Geometry: final body of the model. Coordinates: model frame, mm. A direction names the side the tool comes from. Round coordinates to 2 decimals unless told otherwise and drop trailing zeros. Write each loop counter-clockwise with the first axis right and the second up, starting at its lowest first coordinate (ties: lowest second). Pieces come first, ordered by that corner, then holes. Notation, with made-up numbers: (42, 16) -> (53, 16) arc R27 cw to (53, 47) -> close; hole circle Ø11 at (70, 84). An arc over 180 degrees is marked (long way). Use one line per item in the form item = value. Start each with the question number.
1. Draft query along Y for faces 4 (the face through (35, -37.5, 4)), 5 (the face through (68.217, 35.647, 8.098)), 6 (the face through (70, 0, 8)), 7 (the face through (35.042, -42.571, 17.802)). Return one class per face: pulls with the +Y half, pulls with the -Y half, needs draft (parallel to the pull), parting line crosses it, or undercut.
2. Line query: L1, parallel to Y at x = 27.5, z = 14.75; L2, parallel to X at y = -10, z = 4; L3, parallel to Y at x = -39, z = 13.5. Output: solid intervals per line, ascending.
3. Pin query (flat end, axial travel): pin 1 Ø6 at (x, z) = (-37, 6) entering from +Y; pin 2 Ø1.5 at (x, y) = (19, -17.5) entering from +Z; pin 3 Ø3.5 at (y, z) = (-41, 10) entering from -X; pin 4 Ø1.2 at (y, z) = (-41.5, 15) entering from -X. Return the tip coordinate at first contact, or that it passes through.
4. Cut plane B-B, the plane y = 29. Return the cut outline in (x, z), plus the area to 3 significant figures.
5. Reachability of faces 1 (the face through (-68.681, -35.883, 7.902)), 2 (the face through (1, 37, 8)), 3 (the face through (32, -40, 13)) from +Z, -Z, +X, -X, +Y, -Y: full face, straight path, thin tool, end or side. Return the list, or none.
6. Cut plane C-C, the plane x = -14. Return the cut outline in (y, z).
```python
from build123d import *

# Parameters (mm, degrees)
PAD_DEPTH            = 15
POCKET_DEPTH         = 14
SKETCH002_R          = 1
PAD001_DEPTH         = 140
SKETCH008_W          = 20
SKETCH008_H          = 20
SKETCH008_W_2        = 6
SKETCH008_W_3        = 64
POCKET004_DEPTH      = 15.001
POCKET004_DEPTH_BACK = 3.001
SKETCH009_W          = 15
SKETCH009_H          = 3.5
PAD004_DEPTH         = 1
POCKET005_DEPTH      = 140.001
CHAMFER001_SIZE      = 1


with BuildPart() as part:
    # Sketch → Pad (new body)
    with BuildSketch(Plane.XY):
        with BuildLine():
            Line((-70, 32.5), (-70, -32.5))
            ThreePointArc((-70, -32.5), (-68.535534, -36.035534), (-65, -37.5))
            Line((-65, -37.5), (65, -37.5))
            ThreePointArc((65, -37.5), (68.535534, -36.035534), (70, -32.5))
            Line((70, -32.5), (70, 32.5))
            ThreePointArc((70, 32.5), (68.535534, 36.035534), (65, 37.5))
            Line((65, 37.5), (-65, 37.5))
            ThreePointArc((-65, 37.5), (-68.535534, 36.035534), (-70, 32.5))
        make_face()
    extrude(amount=PAD_DEPTH)

    # Sketch001 (on Face10 of Pad) → Pocket (cut)
    with BuildSketch(Plane.XY.offset(15)):
        with BuildLine():
            Line((-69.5, 32.5), (-69.5, -32.5))
            ThreePointArc((-69.5, -32.5), (-68.181981, -35.681981), (-65, -37))
            Line((-65, -37), (65, -37))
            ThreePointArc((65, -37), (68.181981, -35.681981), (69.5, -32.5))
            Line((69.5, -32.5), (69.5, 32.5))
            ThreePointArc((69.5, 32.5), (68.181981, 35.681981), (65, 37))
            Line((65, 37), (-65, 37))
            ThreePointArc((-65, 37), (-68.181981, 35.681981), (-69.5, 32.5))
        make_face()
    extrude(amount=-POCKET_DEPTH, mode=Mode.SUBTRACT)

    # Sketch002 (on Face9 of Pocket) → Pad001 (join)
    with BuildSketch(Plane.YZ.offset(70)):
        with BuildLine():
            ThreePointArc((-38.5, 15), (-42.64805, 17.771639), (-43.62132, 12.87868))
            Line((-43.62132, 12.87868), (-37.5, 6.757359))
            Line((-37.5, 15), (-37.5, 6.757359))
            Line((-37.5, 15), (-38.5, 15))
        make_face()
        with Locations((-41.5, 15)):
            Circle(SKETCH002_R, mode=Mode.SUBTRACT)
    extrude(amount=-PAD001_DEPTH)

    # Sketch008 (on Face17 of Pad001) → Pocket004 (cut, two sides)
    with BuildSketch(Plane.XY.offset(15)) as pocket004_sk:
        with Locations((-60, -47.49)):
            Rectangle(SKETCH008_W, SKETCH008_H)
        with Locations((60, -47.49)):
            Rectangle(SKETCH008_W, SKETCH008_H)
        with Locations((41, -47.49)):
            Rectangle(SKETCH008_W_2, SKETCH008_H)
        with Locations((-41, -47.49)):
            Rectangle(SKETCH008_W_2, SKETCH008_H)
        with Locations((0, -47.49)):
            Rectangle(SKETCH008_W_3, SKETCH008_H)
    extrude(amount=-POCKET004_DEPTH, mode=Mode.SUBTRACT)
    extrude(pocket004_sk.sketch, amount=POCKET004_DEPTH_BACK, mode=Mode.SUBTRACT)

    # Sketch009 (on Face6 of Pocket004) → Pad004 (join)
    with BuildSketch(Plane(origin=(0, 37.5, 0), x_dir=(-1, 0, 0), z_dir=(0, 1, 0))):
        with Locations((32.5, 12.25)):
            Rectangle(SKETCH009_W, SKETCH009_H)
        with Locations((-32.5, 12.25)):
            Rectangle(SKETCH009_W, SKETCH009_H)
    extrude(amount=PAD004_DEPTH)

    # Sketch010 (on Face1 of Pad004) → Pocket005 (cut, through all)
    with BuildSketch(Plane(origin=(-70, 0, 0), x_dir=(0, -1, 0), z_dir=(-1, 0, 0))):
        Polygon((-37.5, 10.5), (-38.5, 11.5), (-38.5, 10.5), align=None)
        Polygon((-38.5, 13), (-37.5, 14), (-38.5, 14), align=None)
    extrude(amount=-POCKET005_DEPTH, mode=Mode.SUBTRACT)

    # Chamfer001
    chamfer001_edges = [part.edges().sort_by_distance(p)[0] for p in [
        (-68.535534, 36.035534, 0),
        (0, 37.5, 0),
        (68.535534, 36.035534, 0),
        (70, 0, 0),
        (68.645569, -35.921962, 0),
        (57.658035, -37.49, 0),
        (50, -37.495, 0),
        (47, -37.5, 0),
        (44, -37.495, 0),
        (41, -37.49, 0),
        (38, -37.495, 0),
        (35, -37.5, 0),
        (32, -37.495, 0),
        (0, -37.49, 0),
        (-32, -37.495, 0),
        (-35, -37.5, 0),
        (-38, -37.495, 0),
        (-41, -37.49, 0),
        (-44, -37.495, 0),
        (-47, -37.5, 0),
        (-50, -37.495, 0),
        (-57.658035, -37.49, 0),
        (-68.645569, -35.921962, 0),
        (-70, 0, 0),
    ]]
    chamfer(chamfer001_edges, length=CHAMFER001_SIZE)


solid = part.part
```
Outcome:
q1.face_4 = pulls with the -Y half
q1.face_5 = undercut
q1.face_6 = needs draft
q1.face_7 = parting line crosses it
q2.L1 = -37.49 to -37, 37 to 37.5
q2.L2 = -70 to -69.5, 69.5 to 70
q2.L3 = -37.49 to -37, 37 to 38
q3.pin_1 = 37.5
q3.pin_2 = 1
q3.pin_3 = -50
q3.pin_4 = through
q4.outline = (-70, 1) -> (-69, 0) -> (69, 0) -> (70, 1) -> (70, 15) -> (69.5, 15) -> (69.5, 1) -> (-69.5, 1) -> (-69.5, 15) -> (-70, 15) -> close
q4.area = 153 mm^2
q5.face_1 = +Z, -Z, -X, -Y
q5.face_2 = +Z
q5.face_3 = +Z, -Z, -Y
q6.outline = (-37.49, 1) -> (-36.49, 0) -> (36.5, 0) -> (37.5, 1) -> (37.5, 15) -> (37, 15) -> (37, 1) -> (-37, 1) -> (-37, 15) -> (-37.49, 15) -> close
